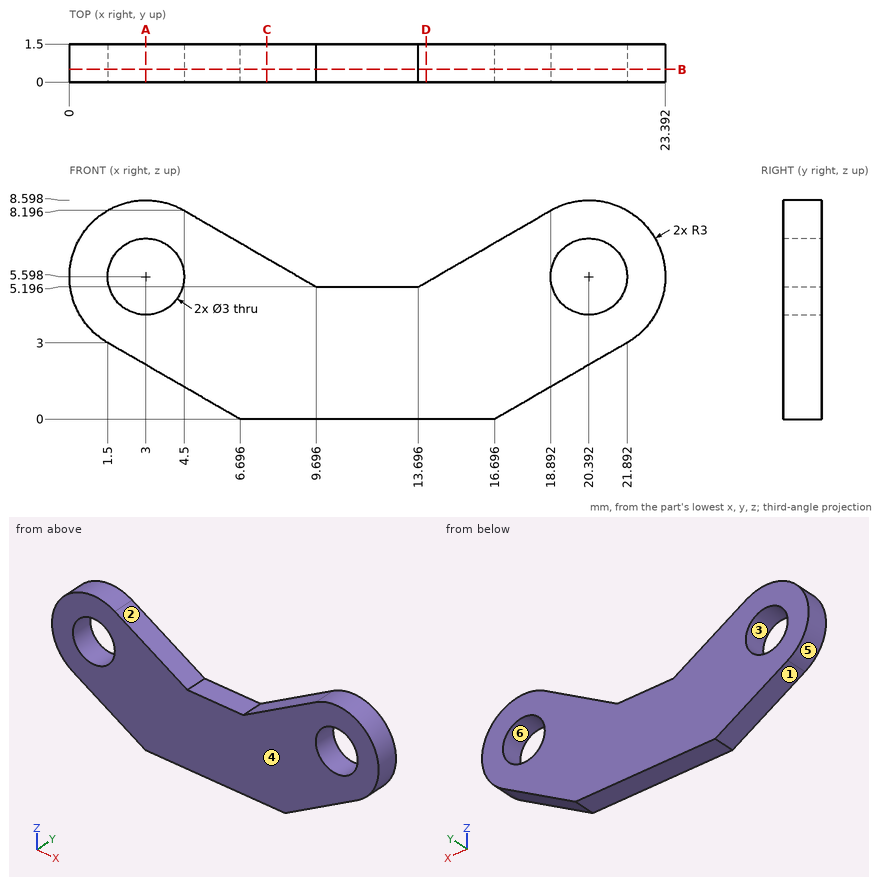
Part print with two shaded views. Sizes in mm from the minimum x, y, z corner. A direction names the side the tool comes from. Coordinates: 2 decimals unless noted, no trailing zeros. Write each loop counter-clockwise with the first axis right and the second up, starting at its lowest first coordinate (ties: lowest second). Pieces come first, ordered by that corner, then holes. Notation, with made-up numbers: (-26, -28) -> (23, -28) arc R15 ccw to (23, -10) -> close; hole circle Ø6 at (34.25, -28.75). An arc over 180 degrees is marked (long way). Return JSON: item names as keys, results as strings. Group by question number.
Q1. Cut at D-D, the plane x = 14. Give the cut face in (y, z).
Q2. Pull direction Z, two halves, no side cores. Call the marked faces 3, 4, 5 and 6: released by +Z, released by -Z, zero draft, split by the parting line, or undercut.
Q3. Drill centre lines: line 1 (X direction, y = 0.7, z = 5.75) (1 decimal); line 2 (X direction, y = 1.05, z = 6) (1 decimal); line 3 (Z direction, x = 12, y = 1.1). Where is each one in solid material? Low to high.
Q4. Cut at C-C, the plane x = 7.75. Give the cut face in (y, z).
Q5. Cut at B-B, the plane y = 0.5. Give the cut face in (x, z).
Q6. Cut at A-A, the plane x = 3. Give the cut face in (y, z).
Q7. Which spindle directions (+Z, -Z, +X, -X, +Y, -Y) get a long thin tool onto all of the face, cutting with end or side? Do the marked faces 1 and 2. Say none if no direction does.
Returned:
{
 "1": {"outline": "(0, 0) -> (1.5, 0) -> (1.5, 5.37) -> (0, 5.37) -> close"},
 "2": {"face 3": "undercut", "face 4": "zero draft", "face 5": "split by the parting line", "face 6": "undercut"},
 "3": {"line 1": "x = 0 to 1.5, 4.5 to 8.7, 14.7 to 18.9, 21.9 to 23.4", "line 2": "x = 0 to 1.6, 4.4 to 8.3, 15.1 to 18.9, 21.8 to 23.4", "line 3": "z = 0 to 5.2"},
 "4": {"outline": "(0, 0) -> (1.5, 0) -> (1.5, 6.32) -> (0, 6.32) -> close"},
 "5": {"outline": "(1.5, 3) -> (6.7, 0) -> (16.7, 0) -> (21.89, 3) arc R3 ccw to (18.89, 8.2) -> (13.7, 5.2) -> (9.7, 5.2) -> (4.5, 8.2) arc R3 ccw to start; hole circle Ø3 at (3, 5.6); hole circle Ø3 at (20.39, 5.6)"},
 "6": {"outline": "(0, 2.13) -> (1.5, 2.13) -> (1.5, 4.1) -> (0, 4.1) -> close; (0, 7.1) -> (1.5, 7.1) -> (1.5, 8.6) -> (0, 8.6) -> close"},
 "7": {"face 1": "-Z, -X, +Y, -Y", "face 2": "+Z, +Y, -Y"}
}
